Geometry: see drawing. Coordinates: mm, zero at the bounding-box minimum. Give positions to 0.01 mm unless a question says otherwise; leave off trailing zeros. Order: outer loops, then holes, each group sorted by start corner. A loop starts at its lowest first (then second) coordinate and runs counter-clockwise, first axis right, second up. Notation, with made-up numbers: (20, 46.5) - (55, 46.5) arc R26 cw to (55, 84.5) - close; hole circle Ø10 at (24.25, 88). An arc over 180 degrees is marked (long way). One line per item, written item: value. Start each with the question number.
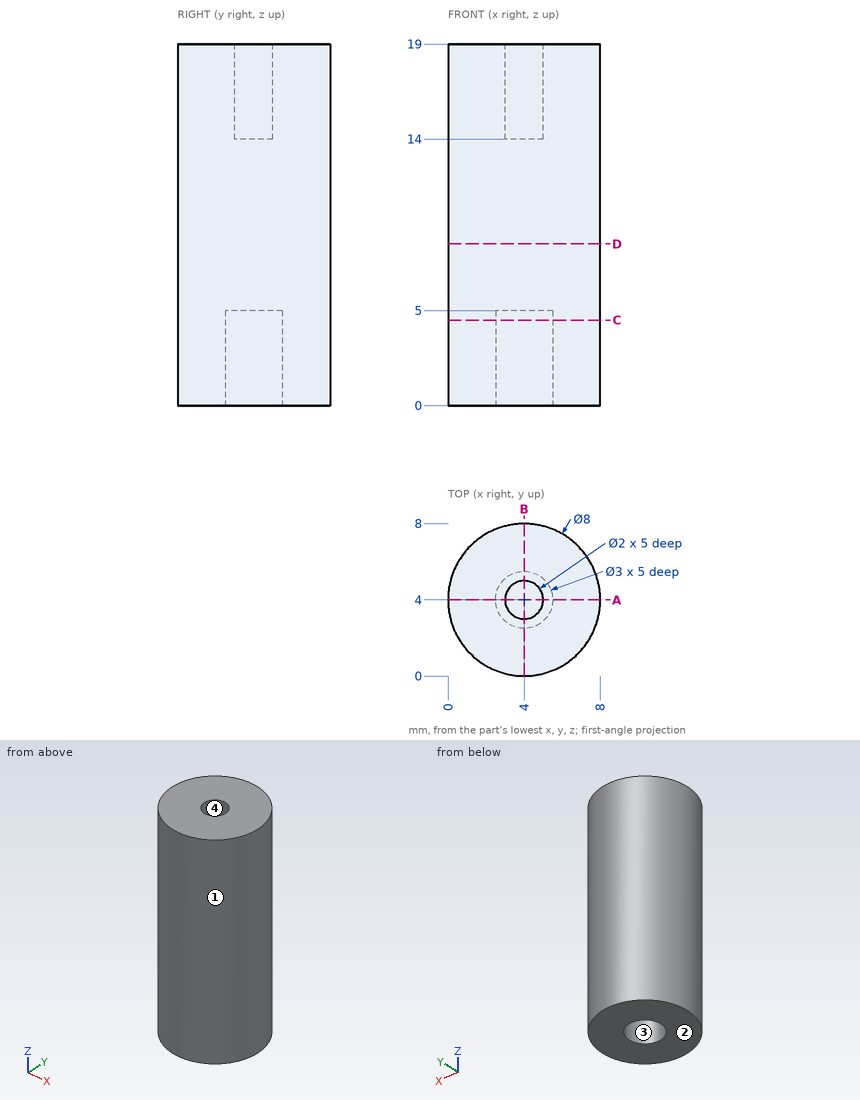
1. Section D-D on z = 8.5. Return the cut outline in (x, y), then the cut area to 3 significant figures.
2. Ray query, L1, parallel to Y at x = 4, z = 17.25; L2, parallel to Z at x = 5.25, y = 4.5; L3, parallel to X at y = 5.75, z = 1. Return the intervals inside material, ascending.
3. Contact query for flat-ended pins moving along their axis: pin 1 Ø0.6 at (x, y) = (3.5, 4) entering from +Z; pin 2 Ø1.5 at (x, y) = (4.5, 4) entering from -Z; pin 3 Ø3 at (x, z) = (1, 5.5) entering from -Y. Output: stop coordinate, or through.
4. Section A-A on y = 4. Return the cut outline in (x, z), then the cut area to 3 significant figures.
5. Section C-C on z = 4.5. Return the cut outline in (x, y), then the cut area to 3 significant figures.
6. Draft query along Y for the marked faces 1, 2, 3 and 4. Return one class per face: pulls with the +Y half, pulls with the -Y half, needs draft (parallel to the pull), parting line crosses it, or undercut.
Data:
1. outline: circle Ø8 at (4, 4)
1. area: 50.3 mm2
2. L1: y = 0 to 3, 5 to 8
2. L2: z = 5 to 19
2. L3: x = 0.4 to 7.6
3. pin 1: stops at z = 14
3. pin 2: stops at z = 5
3. pin 3: stops at y = 0.29
4. outline: (0, 0) - (2.5, 0) - (2.5, 5) - (5.5, 5) - (5.5, 0) - (8, 0) - (8, 19) - (5, 19) - (5, 14) - (3, 14) - (3, 19) - (0, 19) - close
4. area: 127 mm2
5. outline: circle Ø8 at (4, 4); hole circle Ø3 at (4, 4)
5. area: 43.2 mm2
6. face 1: parting line crosses it
6. face 2: needs draft
6. face 3: undercut
6. face 4: undercut
